```python
from build123d import *

# Parameters (mm, degrees)
SKIZZE1_W                       = 100
SKIZZE1_H                       = 55
AUFSATZ_LINEAR_AUSTRAGEN1_DEPTH = 38
SKIZZE2_W                       = 100
SKIZZE2_H                       = 20
SCHNITT_LINEAR_AUSTRAGEN1_DEPTH = 33
SKIZZE4_R                       = 1.5
SCHNITT_LINEAR_AUSTRAGEN2_DEPTH = 66.918510299
SKIZZE5_W                       = 92
SKIZZE5_H                       = 28
SCHNITT_LINEAR_AUSTRAGEN3_DEPTH = 30
SKIZZE6_R                       = 1.5
SCHNITT_LINEAR_AUSTRAGEN4_DEPTH = 81.274528962
VERRUNDUNG1_R                   = 3.5
SKIZZE7_W                       = 28
SKIZZE7_H                       = 15
SCHNITT_LINEAR_AUSTRAGEN5_DEPTH = 14
VERRUNDUNG5_R                   = 3.5


with BuildPart() as part:
    # Skizze1 → Aufsatz-Linear austragen1 (new body)
    with BuildSketch(Plane.XY):
        Rectangle(SKIZZE1_W, SKIZZE1_H)
    extrude(amount=AUFSATZ_LINEAR_AUSTRAGEN1_DEPTH)

    # Skizze2 → Schnitt-Linear austragen1 (cut)
    with BuildSketch(Plane.XY.offset(38)):
        with Locations((0, -17.5)):
            Rectangle(SKIZZE2_W, SKIZZE2_H)
    extrude(amount=-SCHNITT_LINEAR_AUSTRAGEN1_DEPTH, mode=Mode.SUBTRACT)

    # Skizze4 → Schnitt-Linear austragen2 (cut, through all)
    with BuildSketch(Plane.XY.offset(5)):
        with Locations((-10, -19.5)):
            Circle(SKIZZE4_R)
        with Locations((10, -19.5)):
            Circle(SKIZZE4_R)
    extrude(amount=-SCHNITT_LINEAR_AUSTRAGEN2_DEPTH, mode=Mode.SUBTRACT)

    # Skizze5 → Schnitt-Linear austragen3 (cut)
    with BuildSketch(Plane.XZ.offset(7.5)):
        with Locations((0, 21.5)):
            Rectangle(SKIZZE5_W, SKIZZE5_H)
    extrude(amount=-SCHNITT_LINEAR_AUSTRAGEN3_DEPTH, mode=Mode.SUBTRACT)

    # Skizze6 → Schnitt-Linear austragen4 (cut, through all)
    with BuildSketch(Plane.XZ.offset(-22.5)):
        with Locations(Location((-22.5, 21.5, 0), (0, 0, 270))):
            Circle(SKIZZE6_R)
        with Locations(Location((22.5, 21.5, 0), (0, 0, 270))):
            Circle(SKIZZE6_R)
    extrude(amount=-SCHNITT_LINEAR_AUSTRAGEN4_DEPTH, mode=Mode.SUBTRACT)

    # Verrundung1
    verrundung1_edges = [part.edges().sort_by_distance(p)[0] for p in [
        (-46, 7.5, 7.5),
        (-46, 7.5, 35.5),
        (46, 7.5, 35.5),
        (46, 7.5, 7.5),
    ]]
    fillet(verrundung1_edges, radius=VERRUNDUNG1_R)

    # Skizze7 → Schnitt-Linear austragen5 (cut)
    with BuildSketch(Plane.ZY.offset(50)):
        with Locations((21.5, 20)):
            Rectangle(SKIZZE7_W, SKIZZE7_H)
    extrude(amount=-SCHNITT_LINEAR_AUSTRAGEN5_DEPTH, mode=Mode.SUBTRACT)

    # Verrundung5
    verrundung5_edges = [part.edges().sort_by_distance(p)[0] for p in [
        (-46.25, 12.5, 35.5),
        (-46.25, 12.5, 7.5),
    ]]
    fillet(verrundung5_edges, radius=VERRUNDUNG5_R)


solid = part.part
```
CAD build for the part. Positions are in the model's coordinates, mm. A direction names the side the tool comes from. Coordinates: 2 decimals unless noted, no trailing zeros. Order: outer loops, then holes, each group sorted by start corner. A loop starts at its lowest first (then second) coordinate and runs counter-clockwise, first axis right, second up. Notation, with made-up numbers: (-32, 77) - (-5, 77) arc R19 ccw to (-5, 108) - close; hole circle Ø1 at (40.5, 9). An arc over 180 degrees is marked (long way). Use a Markdown table: item, result. Add a question column.
(1) Saw through at C-C (z = 30). Give the cut face in (x, y).
(2) Pull direction X, two halves, no side cores. Call faces 1 (the face through (0, -7.5, 7)), 2 (the face through (50, 6, 19)), 3 (the face through (-36, 25, 21)), 4 (the face through (8.89, -18.49, 2.54)): +X half, -X half, draft (parallel to the pull), parting line (faces both ways), or undercut.
(3) Flat gauge pins, fed straight in: pin 1 (2 mm diameter, centred on x = -31.5, z = 26.5, fed in from -Y); pin 2 (4 mm diameter, centred on y = 25, z = 16.5, fed in from -X); pin 3 (8 mm diameter, centred on x = -39, y = -18.5, fed in from +Z). Where does each tip first touch, or does it go through?
(4) Saw through at A-A (x = 22.5). Give the cut face in (y, z).
(5) Saw through at D-D (z = 21.5). Give the cut face in (x, y).
(6) Drill centre lines: line 1 along Z through (x, y) = (31.5, 22); line 2 along X through (y, z) = (26.35, 21.5); line 3 along X through (y, z) = (26, 21). Where is each one in solid material? Low to high. Write a range as [from, to].
(7) Saw through at B-B (y = -19.5). Give the cut face in (x, z).
(8) Which spindle directions (+Z, -Z, +X, -X, +Y, -Y) get a long thin tool onto all of the face, cutting with end or side? Do faces 5 (the face through (-46, 2, 21)), 6 (the face through (-47.031, 14.024, 8.111)), 7 (the face through (46, 7, 21)). Say none if no direction does.
Solved:
| question | item | result |
|---|---|---|
| 1 | outline | (-50, -7.5) - (-46, -7.5) - (-46, 12.5) - (-50, 12.5) - close; (-36, 22.5) - (46, 22.5) - (46, -7.5) - (50, -7.5) - (50, 27.5) - (-36, 27.5) - close |
| 2 | face 1 | draft |
| 2 | face 2 | +X half |
| 2 | face 3 | -X half |
| 2 | face 4 | undercut |
| 3 | pin 1 | stops at y = 22.5 |
| 3 | pin 2 | stops at x = -36 |
| 3 | pin 3 | stops at z = 5 |
| 4 | outline | (-27.5, 0) - (27.5, 0) - (27.5, 20) - (22.5, 20) - (22.5, 7.5) - (-7.5, 7.5) - (-7.5, 5) - (-27.5, 5) - close; (-7.5, 35.5) - (22.5, 35.5) - (22.5, 23) - (27.5, 23) - (27.5, 38) - (-7.5, 38) - close |
| 5 | outline | (-50, -7.5) - (-46, -7.5) - (-46, 12.5) - (-50, 12.5) - close; (-36, 22.5) - (-24, 22.5) - (-24, 27.5) - (-36, 27.5) - close; (-21, 22.5) - (21, 22.5) - (21, 27.5) - (-21, 27.5) - close; (24, 22.5) - (46, 22.5) - (46, -7.5) - (50, -7.5) - (50, 27.5) - (24, 27.5) - close |
| 6 | line 1 | z = [0, 7.5], [35.5, 38] |
| 6 | line 2 | x = [-36, -24], [-21, 21], [24, 50] |
| 6 | line 3 | x = [-36, -23.91], [-21.09, 21.09], [23.91, 50] |
| 7 | outline | (-50, 0) - (-11.5, 0) - (-11.5, 5) - (-50, 5) - close; (-8.5, 0) - (8.5, 0) - (8.5, 5) - (-8.5, 5) - close; (11.5, 0) - (50, 0) - (50, 5) - (11.5, 5) - close |
| 8 | face 5 | +Y, -Y |
| 8 | face 6 | -X, +Y |
| 8 | face 7 | -Y |
